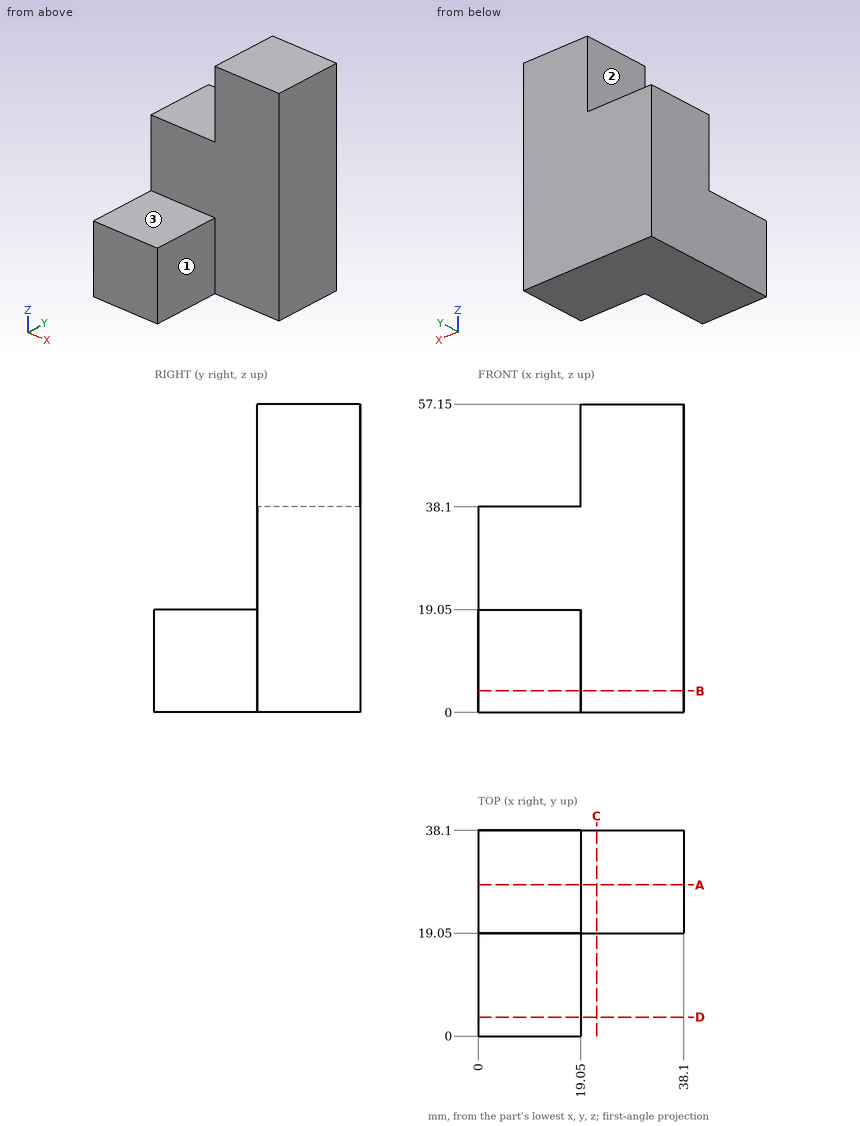
The figure shows three views and two pictorial views of one solid part (mm, origin at its lowest corner). Answer the questions. A direction names the side the tool comes from. Round coordinates to 2 decimals unless told otherwise and drop trailing zeros. Order: outer loops, then holes, each group sorted by start corner. A loop starts at its lowest first (then second) coordinate and runs counter-clockwise, first axis right, second up. Notation, with made-up numbers: (32.25, -19) -> (36.25, -19) arc R17 cw to (36.25, 6) -> close; hole circle Ø2 at (41.5, 47.5). An arc over 180 degrees is marked (long way). One line per item, written item: value.
Item 1: Find section C-C, the plane x = 22. Give the vertices of the cut face in (y, z).
Taken from the geometry:
outline: (19.05, 0) -> (38.1, 0) -> (38.1, 57.15) -> (19.05, 57.15) -> close
Item 2: Given P1, Ø4, axis at x = 15.5, y = 30, coming from the +Z side; P2, Ø10, axis at x = 28.5, z = 14.5, coming from the -Y side; P3, Ø9.5, axis at x = 10.5, y = 14, coming from the +Z side, each flat-ended and moving along its own axis, determine where each tip first touches the part or whether it passes through.
Taken from the geometry:
P1: stops at z = 38.1
P2: stops at y = 19.05
P3: stops at z = 19.05
Item 3: Find section A-A, the plane y = 28. Give the vertices of the cut face in (x, z), then the cut area to 3 significant figures.
Taken from the geometry:
outline: (0, 0) -> (38.1, 0) -> (38.1, 57.15) -> (19.05, 57.15) -> (19.05, 38.1) -> (0, 38.1) -> close
area: 1,810 mm2
Item 4: Find section B-B, the plane z = 4. Give the vertices of the cut face in (x, y).
Taken from the geometry:
outline: (0, 0) -> (19.05, 0) -> (19.05, 19.05) -> (38.1, 19.05) -> (38.1, 38.1) -> (0, 38.1) -> close
Item 5: Straight lines are drawn through the part: L1, parallel to Y at x = 33, z = 28.5; L2, parallel to Z at x = 2, y = 13.5. For each, find the intervals that lie inside material, in ascending order.
Taken from the geometry:
L1: y = 19.05 to 38.1
L2: z = 0 to 19.05
Item 6: For the marked faces 1, 2 and 3, determine the directions among +Z, -Z, +X, -X, +Y, -Y from which every point of the face is accessible in a straight line to the end or side of a thin tool.
Taken from the geometry:
face 1: +Z, -Z, +X, -Y
face 2: +Z, -X, +Y, -Y
face 3: +Z, +X, -X, -Y
Item 7: Find section D-D, the plane y = 3.5. Give the vertices of the cut face in (x, z), then the cut area to 3 significant figures.
Taken from the geometry:
outline: (0, 0) -> (19.05, 0) -> (19.05, 19.05) -> (0, 19.05) -> close
area: 363 mm2
